Autodesk Inventor part; units mm, degrees
ref_plane "YZ Plane" through (0, 0, 0) normal (1, 0, 0) x (0, 1, 0)
ref_plane "XZ Plane" through (0, 0, 0) normal (0, 1, 0) x (-1, 0, 0)
ref_plane "XY Plane" through (0, 0, 0) normal (0, 0, 1) x (1, 0, 0)
sketch "スケッチ1" plane through (0, 0, 0) normal (0, 1, 0) x (-1, 0, 0)
  circle A0 centre (0, 0) radius 178.1675
  circle A1 centre (0, 0) radius 157.8276
  line L0 (168.1877, 0) -> (166.7488, -21.9529)
  line L1 (168.1877, 0) -> (130.1721, 2.4917) construction
  line L2 (249.4344, 0) -> (-249.4344, 0)
  line L3 (166.7488, -21.9529) -> (156.7702, -21.2989)
  line L4 (156.7702, -21.2989) -> (158.2091, 0.654) construction
  line L5 (158.2091, 0.654) -> (168.1877, 0)
  line L6 (157.4896, -10.3224) -> (0, 0)
  line L7 (166.7488, -21.9529) -> (162.4568, -43.5302)
  line L8 (162.4568, -43.5302) -> (152.649, -41.5793) construction
  line L9 (152.649, -41.5793) -> (156.9409, -20.002) construction
  line L10 (156.9409, -20.002) -> (166.7488, -21.9529) construction
  line L11 (162.4568, -43.5302) -> (155.3851, -64.3626)
  line L12 (155.3851, -64.3626) -> (145.9158, -61.1482) construction
  line L13 (145.9158, -61.1482) -> (152.9875, -40.3158) construction
  line L14 (152.9875, -40.3158) -> (162.4568, -43.5302) construction
  line L15 (155.3851, -64.3626) -> (145.6548, -84.0938)
  line L16 (145.6548, -84.0938) -> (136.6861, -79.6709) construction
  line L17 (136.6861, -79.6709) -> (146.4164, -59.9397) construction
  line L18 (146.4164, -59.9397) -> (155.3851, -64.3626) construction
  line L19 (0, 0) -> (111.6009, -111.6009)
  line L20 (145.6548, -84.0938) -> (137.3401, -78.5381) construction
  line L21 (137.3401, -78.5381) -> (125.1176, -96.8305) construction
  line L22 (125.1176, -96.8305) -> (133.4323, -102.3862) construction
  line L23 (133.4323, -102.3862) -> (145.6548, -84.0938)
  line L24 (133.4323, -102.3862) -> (125.9139, -95.7927) construction
  line L25 (125.9139, -95.7927) -> (111.4082, -112.3332) construction
  line L26 (111.4082, -112.3332) -> (118.9266, -118.9266)
  line L27 (118.9266, -118.9266) -> (133.4323, -102.3862)
  line L28 (111.6009, -111.6009) -> (118.9266, -118.9266)
  line L29 (166.7488, -21.9529) -> (176.7274, -22.6069) construction
  line L30 (118.9266, -118.9266) -> (125.9834, -125.9834)
  point P0 (154.795, -30.7906)
  point P1 (149.4517, -50.732)
  point P2 (141.5512, -69.8053)
  point P3 (131.2288, -87.6843)
  point P4 (118.661, -104.0629)
  point P5 (157.8276, 0)
  point P6 (178.1675, 0)
  dimension "d0" = 22
  dimension "d1" = 10
  dimension "d2" = 45
  dimension "d4" = 315.6551
extrude "押し出し1" add sketch "スケッチ1" along normal blind 5.5 contours L30 L27 L23 L15 L11 L7 L0 L2 A0 | L28 A1 L2 L0 L7 L11 L15 L23 L27
sketch "スケッチ2" plane through (0, 5.5, 0) normal (0, 1, 0) x (1, 0, 0)
  circle A0 centre (0, 0) radius 309.8276
  line L0 (-168.1877, 0) -> (-166.7488, 21.9529)
  line L1 (-166.7488, 21.9529) -> (-162.4568, 43.5302)
  line L2 (-162.4568, 43.5302) -> (-155.3851, 64.3626)
  line L3 (-155.3851, 64.3626) -> (-145.6548, 84.0938)
  line L4 (-133.4323, 102.3862) -> (-145.6548, 84.0938)
  line L5 (-118.9266, 118.9266) -> (-133.4323, 102.3862)
  line L6 (-167.4682, 10.9764) -> (-166.0294, 32.9293)
  line L7 (-166.0294, 32.9293) -> (-275.7938, 40.1237)
  line L8 (-275.7938, 40.1237) -> (-277.2327, 18.1708)
  line L9 (-277.2327, 18.1708) -> (-167.4682, 10.9764)
  line L10 (-164.6028, 32.7415) -> (-160.3108, 54.3188)
  line L11 (-160.3108, 54.3188) -> (-268.1972, 75.7787)
  line L12 (-268.1972, 75.7787) -> (-272.4892, 54.2015)
  line L13 (-272.4892, 54.2015) -> (-164.6028, 32.7415)
  circle A1 centre (-166.7488, 21.9529) radius 11
  circle A2 centre (-162.4568, 43.5302) radius 11
  line L14 (-158.921, 53.9464) -> (-151.8493, 74.7789)
  line L15 (-151.8493, 74.7789) -> (-256.0116, 110.1372)
  line L16 (-256.0116, 110.1372) -> (-263.0833, 89.3047)
  line L17 (-263.0833, 89.3047) -> (-158.921, 53.9464)
  circle A3 centre (-155.3851, 64.3626) radius 11
  arc A4 (-275.7591, 62.4834) -> (-281.3553, 41.7349) centre (-166.7488, 21.9529) ccw
  line L18 (-178.1663, 0.654) -> (-158.2091, -0.654)
  line L19 (-158.2091, -0.654) -> (-156.7702, 21.2989)
  line L20 (-156.7702, 21.2989) -> (-176.7274, 22.6069)
  line L21 (-176.7274, 22.6069) -> (-178.1663, 0.654)
  line L22 (-177.4468, 11.6305) -> (-275.7938, 40.1237)
  line L23 (-176.7274, 22.6069) -> (-176.008, 33.5834)
  line L24 (-176.008, 33.5834) -> (-275.7591, 62.4834)
  line L25 (-275.7938, 40.1237) -> (-281.3553, 41.7349)
  circle A5 centre (0, 0) radius 137.8276
  line L26 (0, 0) -> (-219.0812, 219.0812)
  line L27 (-111.6009, 111.6009) -> (-125.9834, 125.9834)
  line L28 (-433.7586, 0) -> (433.7586, 0)
  circle A6 centre (0, 0) radius 279.8276 construction
  arc A7 (-111.6009, 111.6009) -> (-157.8276, 0) centre (0, 0) ccw
  point P0 (-158.1662, 0)
  point P1 (-137.8276, 0)
  point P2 (-97.4588, 97.4588)
  point P3 (-309.8276, 0)
  dimension "d7" = 22
  dimension "d10" = 20
  dimension "d11" = 100
  dimension "d12" = 30
  dimension "d14" = 20
  dimension "d17" = 122
extrude "押し出し2" add sketch "スケッチ2" against normal blind 5.5 contours L26 L5 L4 L3 A3 L15 L16 L17 A2 L11 L12 L24 A4 L25 L8 L9 L21 L18 L28 A0 | L18 L21 L9 L0 | L0 A1 L19 L28 | A5 L28 A7 A1 A2 A3 L26 | L26 A7 A3 L3 L4 L5 | A1 L21 L20 L0 | L9 L21 A1 | L0 L20 L19 A1 | L19 A7 L28 | L6 A1 L1 | L20 L23 A1 L6 | L1 A1 A7 L19 L20 | L22 L7 L23 A1 L21 | L9 L8 L22 | A1 L23 L21 | A1 A7 L19 | A7 A3 L2 L3 | A3 A7 | A2 L10 L1 | A1 L7 L24 L13 | A2 A7 A1 | L13 L24 L12 L11 A2 | L1 L2 A2 A7 | A1 L23 L7 | L25 A4 L24 L12 L13 L7 | A7 A1 | A7 A2 A3 | L3 L14 A3 | L10 A2 L2 | L13 L12 L24 | A7 A2 | A3 L14 L2 | L17 L16 L15 A3
sketch "スケッチ3" plane through (0, 5.5, 0) normal (0, 1, 0) x (1, 0, 0)
  circle A0 centre (0, 0) radius 289.8276
  arc A1 (-97.4588, 97.4588) -> (-137.8276, 0) centre (0, 0) ccw
  line L0 (-97.4588, 97.4588) -> (-219.0812, 219.0812)
  line L1 (-309.8276, 0) -> (-137.8276, 0)
  arc A2 (-219.0812, 219.0812) -> (-309.8276, 0) centre (0, 0) ccw
  point P0 (-289.8276, 0)
  point P1 (-204.939, 204.939)
  dimension "d21" = 20
extrude "押し出し3" cut sketch "スケッチ3" against normal through all contours L0 A1 L1 A0 picked at (-207.353, 118.7807)
sketch "スケッチ4" plane through (0, 5.5, 0) normal (0, 1, 0) x (1, 0, 0)
  circle A0 centre (-299.8276, 4.7) radius 1.6
  line L0 (-304.8276, 34.2) -> (-294.8276, 34.2)
  line L1 (-294.8276, 34.2) -> (-294.8276, 31.2)
  line L2 (-294.8276, 31.2) -> (-304.8276, 31.2)
  line L3 (-304.8276, 31.2) -> (-304.8276, 34.2)
  line L4 (-301.3276, 37.7) -> (-298.3276, 37.7)
  line L5 (-298.3276, 37.7) -> (-298.3276, 27.7)
  line L6 (-298.3276, 27.7) -> (-301.3276, 27.7)
  line L7 (-301.3276, 27.7) -> (-301.3276, 37.7)
  line L8 (-309.8276, 0) -> (-289.8276, 0)
  line L9 (0, 0) -> (-215.9005, 89.4289) construction
  line L10 (-371.7931, 0) -> (61.9655, 0)
  circle A1 centre (-215.3335, 208.6867) radius 1.6
  line L11 (-239.7287, 191.3626) -> (-232.6576, 184.2915)
  line L12 (-232.6576, 184.2915) -> (-230.5363, 186.4128)
  line L13 (-230.5363, 186.4128) -> (-237.6074, 193.4839)
  line L14 (-237.6074, 193.4839) -> (-239.7287, 191.3626)
  line L15 (-239.7287, 186.4128) -> (-237.6074, 184.2915)
  line L16 (-237.6074, 184.2915) -> (-230.5363, 191.3626)
  line L17 (-230.5363, 191.3626) -> (-232.6576, 193.4839)
  line L18 (-232.6576, 193.4839) -> (-239.7287, 186.4128)
  line L19 (-219.0812, 219.0812) -> (-204.939, 204.939)
  point P0 (-294.8276, 32.7)
  point P1 (-298.3276, 32.7)
  point P2 (-299.8276, 37.7)
  point P3 (-299.8276, 34.2)
  point P4 (-299.8276, 27.7)
  point P5 (-299.8276, 0)
  point P6 (-299.8276, 0)
  point P7 (-231.597, 185.3522)
  point P8 (-234.0718, 187.8271)
  point P9 (-238.668, 185.3522)
  point P10 (-236.1932, 187.8271)
  point P11 (-231.597, 192.4232)
  point P12 (-212.0101, 212.0101)
  point P13 (-212.0101, 212.0101)
  point P14 (-301.3276, 34.2)
  point P15 (-301.3276, 31.2)
  point P16 (-298.3276, 31.2)
  point P17 (-298.3276, 34.2)
  point P18 (-233.0112, 188.8877)
  point P19 (-235.1325, 191.009)
  point P20 (-237.2538, 188.8877)
  point P21 (-235.1325, 186.7664)
  dimension "d22" = 3
  dimension "d23" = 10
  dimension "d24" = 27.7
  dimension "d25" = 4.7
  dimension "d26" = 3.2
  dimension "d27" = 22.5
extrude "押し出し4" cut sketch "スケッチ4" against normal through all
properties part number "front_under" material "木材 (カエデ材)"
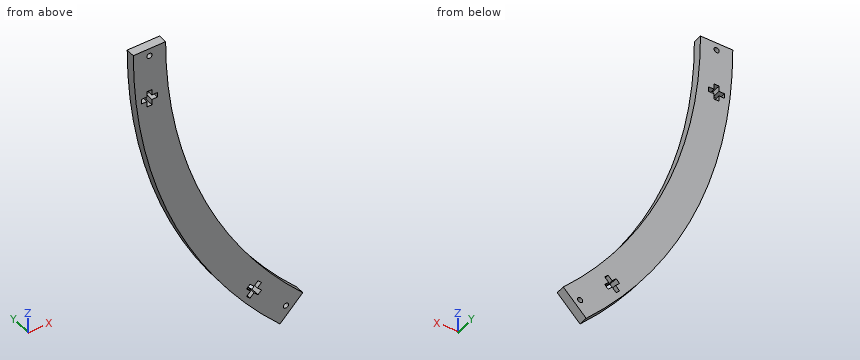
Check sheet for the modelled part. Datum: model origin and axes. Units: mm. Give positions to 0.01 mm unless a question says otherwise; leave off trailing zeros. Write each loop counter-clockwise with the first axis right and the second up, starting at its lowest first coordinate (ties: lowest second). Pieces come first, ordered by that corner, then holes.
Item 1: Scan lines: L1, parallel to X at y = 2.05, z = -185; L2, parallel to X at y = 2.2, z = -4.7; L3, parallel to Z at x = -236, y = 1.95. Record each from-to range of solid material in increasing order.
Item 2: Cross-section at B-B (z = -144). Enter the section's corners in (x, y).
Item 3: Cross-section at A-A (y = 4.6). Count the separate pieces of the cut face and the enclosed holes in it, and give its area (3 significant figures).
Item 4: Cross-section at C-C (x = -282.5). Enter the section's corners in (y, z).
Item 5: Gauge pin test, flat ends, axial feed: pin 1 (1.5 mm diameter, centred on y = 4.5, z = -24.5, fed in from +X); pin 2 (1.8 mm diameter, centred on y = 3.5, z = -29.5, fed in from +X); pin 3 (3 mm diameter, centred on y = 2.5, z = -35.5, fed in from +X). Record the tip position at first contact, or that the pin passes through.
Report:
1. L1: x = -248.53 to -238.32, -236.9 to -233.37, -231.95 to -223.1
1. L2: x = -309.79 to -301.43, -298.23 to -289.79
1. L3: z = -200.74 to -191.88, -185.9 to -168.24
2. outline: (-274.33, 0) - (-251.52, 0) - (-251.52, 5.5) - (-274.33, 5.5) - close
3. separate pieces: 1
3. enclosed holes: 4
3. area: 4,590 mm2
4. outline: (0, -127.23) - (5.5, -127.23) - (5.5, -64.76) - (0, -64.76) - close
5. pin 1: stops at x = -288.73
5. pin 2: stops at x = -288.23
5. pin 3: stops at x = -287.46
